from build123d import *

# Parameters (mm, degrees)
F0_R      = 11.75
F3_DEPTH  = 28
F4_R      = 5.25
F5_DEPTH  = 14
F2_R      = 3.2
F6_DEPTH  = 14
F7_W      = 5.7
F7_H      = 2.7
F8_DEPTH  = 9
F9_W      = 5.7
F9_H      = 2.6
F10_DEPTH = 9
F11_R     = 1.5
F12_DEPTH = 25
F13_R     = 1.5
F14_DEPTH = 25


with BuildPart() as f3:
    # F0 (on Top) → F3 (new body)
    with BuildSketch(Plane.XY):
        Circle(F0_R)
    extrude(amount=F3_DEPTH)

    # F4 (on Top) → F5 (cut)
    with BuildSketch(Plane.XY):
        Circle(F4_R)
    extrude(amount=F5_DEPTH, mode=Mode.SUBTRACT)

    # F2 (on offset) → F6 (cut)
    with BuildSketch(Plane.XY.offset(28)):
        Circle(F2_R)
    extrude(amount=-F6_DEPTH, mode=Mode.SUBTRACT)

    # F7 (on offset) → F8 (cut)
    with BuildSketch(Plane.XY.offset(28)):
        with Locations((0, 5.35)):
            Rectangle(F7_W, F7_H)
    extrude(amount=-F8_DEPTH, mode=Mode.SUBTRACT)

    # F9 (on Top) → F10 (cut)
    with BuildSketch(Plane.XY):
        with Locations((0, -7.35)):
            Rectangle(F9_W, F9_H)
    extrude(amount=F10_DEPTH, mode=Mode.SUBTRACT)

    # F11 (on Front) → F12 (cut)
    with BuildSketch(Plane.XZ):
        with Locations((0, 4.5)):
            Circle(F11_R)
    extrude(amount=F12_DEPTH, mode=Mode.SUBTRACT)

    # F13 (on Front) → F14 (cut)
    with BuildSketch(Plane.XZ):
        with Locations((0, 23.5)):
            Circle(F13_R)
    extrude(amount=-F14_DEPTH, mode=Mode.SUBTRACT)


solid = f3.part
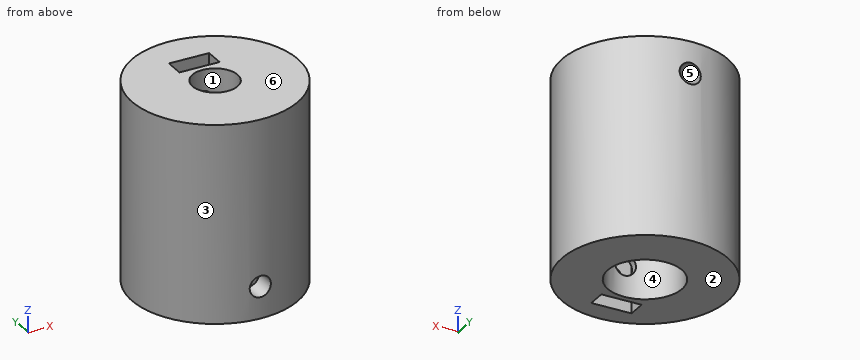
Part model, mm, in its own coordinate system. Face numbers are marked on the shaded views. A direction names the side the tool comes from. Coordinates: 2 decimals unless noted, no trailing zeros. Loops run counter-clockwise (first coordinate to the right, second up) from the corner with the lowest first, then second, coordinate; pieces in that order, holes last. Notation, with made-up numbers: M 69,16.5 L 100,16.5 A29 cw 100,40.5 Z; hole C 80.5,-36.75 d5. An arc over 180 degrees is marked long. Use a Markdown table: item, result. Add a question column.
Q1. Pin check, flat tips, straight feed: P1, Ø2.5, axis at x = 0, z = 4.5, coming from the -Y side; P2, Ø1.3, axis at x = 0, y = -7.5, coming from the -Z side; P3, Ø1.3, axis at y = -7, z = 6.5, coming from the +X side. Stop position of each tip, or through.
Q2. Mould opens along X. For the marked faces 1, 2 and 3 say: +X half, -X half, draft (parallel to the pull), parting line (faces both ways), or undercut.
Q3. Probe L1, parallel to Y at x = 0, z = 7.75; L2, parallel to Z at x = 0, y = -5.55; L3, parallel to Z at x = 0, y = 8.5. List the from-to ranges inside material, lowest first.
Q4. Cut at B-B (z = 4.5). Write the cut outline in (x, y).
Q5. Cut at C-C (x = 0). Give the number of separate pieces and of enclosed holes in the cut face, and give its area (3 significant figures).
Q6. Which spindle directions (+Z, -Z, +X, -X, +Y, -Y) get a long thin tool onto all of the face, cutting with end or side? Do the marked faces 4, 5 and 6. Say none if no direction does.
Q7. Cut at D-D (y = 9.75). Write the cut outline in (x, z), and give its area (3 significant figures).
Q8. Cut at A-A (y = 0). Write the cut outline in (x, z), and give its area (3 significant figures).
Worked out:
| question | item | result |
|---|---|---|
| 1 | P1 | stops at y = 5.1 |
| 1 | P2 | stops at z = 9 |
| 1 | P3 | stops at x = 9.89 |
| 2 | face 1 | undercut |
| 2 | face 2 | draft |
| 2 | face 3 | parting line |
| 3 | L1 | y = -11.75 to -8.65, -6.05 to -5.25, 5.25 to 11.75 |
| 3 | L2 | z = 0 to 3, 6 to 28 |
| 3 | L3 | z = 0 to 22, 25 to 28 |
| 4 | outline | M -2.85,-8.65 L -2.85,-6.05 L -1.5,-6.05 L -1.5,-5.03 A5.25 cw long 1.5,-5.03 L 1.5,-6.05 L 2.85,-6.05 L 2.85,-8.65 L 1.5,-8.65 L 1.5,-11.65 A11.75 ccw long -1.5,-11.65 L -1.5,-8.65 Z |
| 5 | separate pieces | 6 |
| 5 | enclosed holes | 0 |
| 5 | area | 344 mm2 |
| 6 | face 4 | -Z |
| 6 | face 5 | +Y |
| 6 | face 6 | +Z, +X, -X, +Y, -Y |
| 7 | outline | M -6.56,0 L 6.56,0 L 6.56,28 L -6.56,28 Z; hole C 0,23.5 d3 |
| 7 | area | 360 mm2 |
| 8 | outline | M -11.75,0 L -5.25,0 L -5.25,14 L -3.2,14 L -3.2,28 L -11.75,28 Z; M 3.2,14 L 5.25,14 L 5.25,0 L 11.75,0 L 11.75,28 L 3.2,28 Z |
| 8 | area | 421 mm2 |
